Design review of the part built by this model. Coordinates are the model's own, in mm. A direction names the side the tool comes from. Round coordinates to 2 decimals unless told otherwise and drop trailing zeros. Loops run counter-clockwise (first coordinate to the right, second up) from the corner with the lowest first, then second, coordinate; pieces in that order, holes last. Notation, with made-up numbers: (61.25, 27) - (96.25, 27) arc R22 ccw to (96.25, 38) - close; hole circle Ø1 at (44, 54.25). An arc over 180 degrees is marked (long way). Return JSON: item names as keys, results as strings. Group by question number.
(1) We need section D-D, the plane y = -4.75. Write out the cut boundary in (x, z) (1 decimal).
(2) We need section A-A, the plane x = 0. Write out the cut boundary in (y, z).
(3) For faces 4 (the conical face through (1.148, -5.653, -2.206)), 5 (the flat face through (0, 3, 0)), list the 3-axis set-ups (+Z, -Z, +X, -X, +Y, -Y) from which the entire face can be reached by the end or side of a thin tool; tool diameter is ignored.
(4) Clearance check with a flat-ended pin moving along its axis: pin 1 (2 mm diameter, centred on y = 5, z = 1.5, fed in from +X). State where the tip first meets the part, or that it passes through.
(5) We need section B-B, the plane y = 3. Write out the cut boundary in (x, z), and give its area (3 significant figures).
(6) The part is to be moulded in two halves that separate along Y. For faces 1 (the cylindrical face through (-1.6, 1.8, 1.4)), 2 (the flat face through (0, -6, 0)), 3 (the flat face through (0, 6, 0)), say which applies: pulls with the +Y half, pulls with the -Y half, needs draft (parallel to the pull), parting line crosses it, or undercut.
(7) Wall thickness on L1, parallel to Y at x = 0, z = 1.7; L2, parallel to X at y = 3, z = 0.9; L3, parallel to Y at x = 0.9, z = 1.5: over which ranges is each line inside the solid? List them lowest first. Write a range as [from, to].
(8) We need section C-C, the plane y = 0.75. Write out the cut boundary in (x, z), and give its area (3 significant figures).
from build123d import *

# Parameters (mm, degrees)
F0_R     = 2.9
F1_DEPTH = 6
F2_R     = 2
F3_DEPTH = 2.9
F4_SIZE2 = 2
F4_SIZE  = 0.5


with BuildPart() as f1:
    # F0 (on Front) → F1 (new body, symmetric)
    with BuildSketch(Plane.XZ):
        Circle(F0_R)
    extrude(amount=F1_DEPTH, both=True)

    # F2 (on Top) → F3 (cut, through all)
    with BuildSketch(Plane.XY):
        with Locations((0, 3)):
            Circle(F2_R)
    extrude(amount=F3_DEPTH, mode=Mode.SUBTRACT)

    # F4
    f4_edges = [f1.edges().sort_by_distance(p)[0] for p in [
        (-2.9, -6, 0),
    ]]
    f4_side = f1.faces().sort_by_distance((0, -6, 0))[0]
    chamfer(f4_edges, length=F4_SIZE, length2=F4_SIZE2, reference=f4_side)


solid = f1.part
Solutions:
{
 "1": {"outline": "circle Ø5.4 at (0, 0)"},
 "2": {"outline": "(-6, -2.4) - (-4, -2.9) - (6, -2.9) - (6, 2.9) - (5, 2.9) - (5, 0) - (1, 0) - (1, 2.9) - (-4, 2.9) - (-6, 2.4) - close"},
 "3": {"face 4": "-Y", "face 5": "+Z"},
 "4": {"pin 1": "x = 2.86"},
 "5": {"outline": "(-2, 0) - (-2, 2.1) arc R2.9 ccw (long way) to (2, 2.1) - (2, 0) - close", "area": "15.8 mm^2"},
 "6": {"face 1": "undercut", "face 2": "pulls with the -Y half", "face 3": "pulls with the +Y half"},
 "7": {"L1": "[-6, 1], [5, 6]", "L2": "[-2.76, -2], [2, 2.76]", "L3": "[-6, 1.21], [4.79, 6]"},
 "8": {"outline": "circle Ø5.8 at (0, 0)", "area": "26.4 mm^2"}
}
